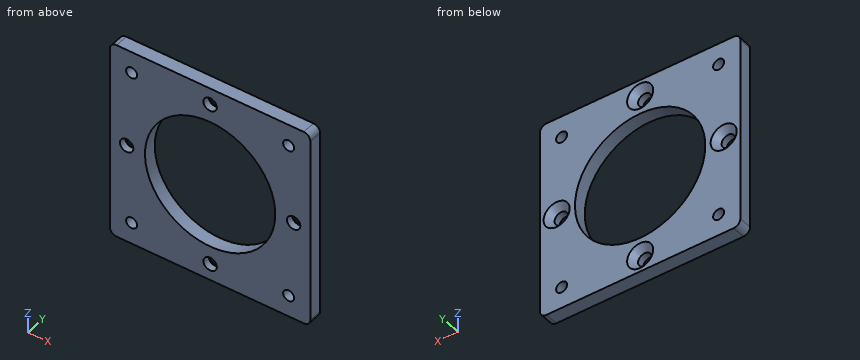
from build123d import *

# Parameters (mm, degrees)
SKETCH_1_W      = 60
SKETCH_1_H      = 60
SKETCH_1_R      = 1.65
SKETCH_1_R_2    = 19.5
SKETCH_1_R_3    = 2
EXTRUDE_1_DEPTH = 4
FILLET_1_R      = 2
CHAMFER_1_SIZE  = 1.9


with BuildPart() as part:
    # Эскиз1 → Бобышка-Вытянуть1 (new body)
    with BuildSketch(Plane(origin=(0, 0, 0), x_dir=(1, 0, 0), z_dir=(0, 1, 0))):
        with Locations((-9.094903125, 3.781032797)):
            Rectangle(SKETCH_1_W, SKETCH_1_H)
        with Locations(Location((-32.594903125, 27.281032797, 0), (0, 0, 270))):
            Circle(SKETCH_1_R, mode=Mode.SUBTRACT)
        with Locations(Location((14.405096875, 27.281032797, 0), (0, 0, 270))):
            Circle(SKETCH_1_R, mode=Mode.SUBTRACT)
        with Locations(Location((-32.594903125, -19.718967203, 0), (0, 0, 270))):
            Circle(SKETCH_1_R, mode=Mode.SUBTRACT)
        with Locations(Location((14.405096875, -19.718967203, 0), (0, 0, 270))):
            Circle(SKETCH_1_R, mode=Mode.SUBTRACT)
        with Locations(Location((-9.094903125, 3.781032797, 0), (0, 0, 270))):
            Circle(SKETCH_1_R_2, mode=Mode.SUBTRACT)
        with Locations(Location((-34.094903125, 3.781032797, 0), (0, 0, 270))):
            Circle(SKETCH_1_R_3, mode=Mode.SUBTRACT)
        with Locations(Location((15.905096875, 3.781032797, 0), (0, 0, 270))):
            Circle(SKETCH_1_R_3, mode=Mode.SUBTRACT)
        with Locations(Location((-9.094903125, 28.781032797, 0), (0, 0, 270))):
            Circle(SKETCH_1_R_3, mode=Mode.SUBTRACT)
        with Locations(Location((-9.094903125, -21.218967203, 0), (0, 0, 270))):
            Circle(SKETCH_1_R_3, mode=Mode.SUBTRACT)
    extrude(amount=EXTRUDE_1_DEPTH)

    # Скругление1
    fillet_1_edges = [part.edges().sort_by_distance(p)[0] for p in [
        (-39.094903125, 2, -33.781032797),
        (20.905096875, 2, -33.781032797),
        (20.905096875, 2, 26.218967203),
        (-39.094903125, 2, 26.218967203),
    ]]
    fillet(fillet_1_edges, radius=FILLET_1_R)

    # Фаска1
    chamfer_1_edges = [part.edges().sort_by_distance(p)[0] for p in [
        (-34.094903125, 4, -5.781032797),
        (15.905096875, 4, -5.781032797),
        (-9.094903125, 4, -30.781032797),
        (-9.094903125, 4, 19.218967203),
    ]]
    chamfer(chamfer_1_edges, length=CHAMFER_1_SIZE)


solid = part.part
Part model, mm, in its own coordinate system. Coordinates: 2 decimals unless noted, no trailing zeros. Loops run counter-clockwise (first coordinate to the right, second up) from the corner with the lowest first, then second, coordinate; pieces in that order, holes last. Notation, with made-up numbers: (40.25, -29) - (44.25, -29) arc R22 ccw to (44.25, -12) - close; hole circle Ø9 at (67, 3.5). An arc over 180 degrees is marked (long way). Write each question's results on one line, items separated by ' | '. Start each with the question number.
Q1. Slice it at C-C on y = 2.9. Give the number of separate pieces and of enclosed holes in the cut face, and give its area (3 significant figures).
Q2. Probe line 1 along Z through (x, y) = (14, 3.35); line 2 along X through (y, z) = (2, -26); line 3 along X through (y, z) = (1.9, -28). List the from-to ranges inside material, lowest first.
Q3. Slice it at A-A on x = 3. Give the cut face in (y, z), and give its area (3 significant figures).
Q4. Slice it at B-B on z = -20. Give the cut face in (x, y).
Answer:
1) separate pieces: 1 | enclosed holes: 9 | area: 2,270 mm2
2) line 1: z = -33.78 to -28.88, -25.68 to -6.41, -1.15 to 18.12, 21.32 to 26.22 | line 2: x = -39.09 to -33.63, -31.55 to 13.37, 15.45 to 20.91 | line 3: x = -39.09 to -34.08, -31.11 to -10.94, -7.25 to 12.92, 15.89 to 20.91
3) outline: (0, -33.78) - (4, -33.78) - (4, -19.08) - (0, -19.08) - close; (0, 11.51) - (4, 11.51) - (4, 26.22) - (0, 26.22) - close | area: 118 mm2
4) outline: (-39.09, 0) - (-19.92, 0) - (-19.92, 4) - (-39.09, 4) - close; (1.73, 0) - (20.91, 0) - (20.91, 4) - (1.73, 4) - close
